Geometry check sheet. Reference: the model listing, model coordinates, mm. A direction names the side the tool comes from. Coordinates: 2 decimals unless noted, no trailing zeros. Loops run counter-clockwise (first coordinate to the right, second up) from the corner with the lowest first, then second, coordinate; pieces in that order, holes last.
Autodesk Inventor part; units mm, degrees
ref_plane "YZ Plane" through (0, 0, 0) normal (1, 0, 0) x (0, 1, 0)
ref_plane "XZ Plane" through (0, 0, 0) normal (0, 1, 0) x (-1, 0, 0)
ref_plane "XY Plane" through (0, 0, 0) normal (0, 0, 1) x (1, 0, 0)
sketch "Sketch1" plane through (0, 0, 0) normal (0, 0, 1) x (1, 0, 0)
  line L0 (0, 0) -> (30, 0)
  arc A0 (122.3584, -3.6921) -> (30, 0) centre (76.2499, -0.076) ccw
  line L1 (122.3584, -3.6921) -> (154.7584, -3.6921)
  line L2 (154.7584, -3.6921) -> (357.7584, -3.6921) construction
  line L3 (0, 0) -> (0, 35)
  arc A1 (181.6354, 197.5208) -> (104.7506, 210.6385) centre (143.2612, 204.4794) ccw
  line L4 (122.3584, -3.6921) -> (132.3584, -3.6921)
  line L5 (0, 35) -> (104.7506, 210.6385)
  line L6 (154.7584, -3.6921) -> (181.9168, 199.3079)
  dimension "d0" = 30
  dimension "d1" = 92.5
  dimension "d2" = 32.4
  dimension "d3" = 203
  dimension "d5" = 35
  dimension "d7" = 10
  dimension "d9" = 78
  dimension "d10" = 203
sketch "Sketch2" plane through (0, 0, 0) normal (0, 0, 1) x (1, 0, 0)
  point P0 (0, 0)
extrude "Extrusion1" add sketch "Sketch1" along normal blind 15.3
sketch "Sketch3" plane through (0, 0, 15.3) normal (0, 0, 1) x (1, 0, 0)
  line L0 (154.7584, -3.6921) -> (181.9168, 199.3079)
  arc A0 (94.1987, 192.9457) -> (177.6835, 167.6655) centre (143.2612, 204.4794) ccw
  arc A1 (181.9168, 199.3079) -> (104.7506, 210.6385) centre (143.2612, 204.4794) ccw
  line L1 (104.7506, 210.6385) -> (94.1987, 192.9457)
  line L2 (104.7506, 210.6385) -> (0, 35)
  line L3 (181.9168, 199.3079) -> (177.6835, 167.6655)
  arc A2 (181.9168, 199.3079) -> (104.7506, 210.6385) centre (143.2612, 204.4794) ccw
  point P0 (0, 0)
  dimension "d19" = 100.8
extrude "Extrusion2" add sketch "Sketch3" along normal blind 6
properties part number "volante conjunto"
(1) Sectioned sample at A-A on x = 138.5. Record the cut outline in (y, z).
Findings:
outline: (-3.69, 0) - (243.19, 0) - (243.19, 21.3) - (154.3, 21.3) - (154.3, 15.3) - (-3.69, 15.3) - close
(2) Sectioned sample at D-D on x = 43. Record the cut outline in (y, z).
Findings:
outline: (32.07, 0) - (107.1, 0) - (107.1, 15.3) - (32.07, 15.3) - close
(3) Access from +Z, -Z, +X, -X, +Y, -Y to the whole of each face (thin tool, end or side, straight path). Record for faces 5 (the flat face through (15, 0, 8)), 6 (the flat face through (138, 199, 21.3)).
Findings:
face 5: +Z, -Z, -X, -Y
face 6: +Z, +X, -X, +Y, -Y
(4) Gauge pin test, flat ends, axial feed: pin 1 Ø7.5 at (x, z) = (9, 4.5) entering from -Y; pin 2 Ø6 at (x, y) = (130.5, 90.5) entering from +Z; pin 3 Ø2 at (y, z) = (199.5, 10.5) entering from +X. Record the tip position at first contact, or that the pin passes through.
Findings:
pin 1: stops at y = 0
pin 2: stops at z = 15.3
pin 3: stops at x = 182.06
(5) Draft check along X on faces 1 (the cylindrical face through (77.056, 46.167, 7.543)), 2 (the flat face through (138, -3.692, 8)), 3 (the cylindrical face through (129.362, 156.034, 18.258)), 4 (the flat face through (168.147, 96.387, 8.134)). Enter one of: +X half, -X half, draft (parallel to the pull), parting line (faces both ways), or undercut.
Findings:
face 1: undercut
face 2: draft
face 3: parting line
face 4: +X half
(6) Sectioned sample at B-B on z = 8. Record the cut outline in (x, y).
Findings:
outline: (0, 0) - (30, 0) arc R46.25 cw (long way) to (122.36, -3.69) - (154.76, -3.69) - (181.92, 199.31) arc R39 ccw to (104.75, 210.64) - (0, 35) - close
(7) Sectioned sample at C-C on y = 206.5. Record the cut outline in (x, z), and give its area (3 significant figures).
Findings:
outline: (102.28, 0) - (182.21, 0) - (182.21, 21.3) - (102.28, 21.3) - close
area: 1,700 mm2
(8) Scan lines: L1, parallel to Z at x = 108, y = 66.5; L2, parallel to X at y = 127.5, z = 3; L3, parallel to Y at x = 83, z = 14.75. Record each from-to range of solid material in increasing order.
Findings:
L1: z = 0 to 15.3
L2: x = 55.17 to 172.31
L3: y = 45.68 to 174.17
